Part model, mm, in its own coordinate system. A direction names the side the tool comes from. Coordinates: 2 decimals unless noted, no trailing zeros. Write each loop counter-clockwise with the first axis right and the second up, starting at its lowest first coordinate (ties: lowest second). Pieces come first, ordered by that corner, then holes. Notation, with made-up numbers: (1, -37) - (21, -37) arc R17 ccw to (21, -14) - close; hole circle Ø4 at (19.25, 14). An arc over 180 degrees is marked (long way). Use a Markdown table: item, result.
```python
from build123d import *

# Parameters (mm, degrees)
SKETCH1_W           = 900
SKETCH1_H           = 50
BOSS_EXTRUDE1_DEPTH = 200
BOSS_EXTRUDE2_START = -82
SKETCH4_R           = 20
SKETCH4_R_2         = 15.875
BOSS_EXTRUDE2_DEPTH = 36
SKETCH8_W           = 25
SKETCH8_H           = 252.75
BOSS_EXTRUDE3_DEPTH = 25
FILLET1_R           = 50
SKETCH9_R           = 15.875
BOSS_EXTRUDE4_DEPTH = 18


with BuildPart() as part:
    # Sketch1 → Boss-Extrude1 (new body)
    with BuildSketch(Plane.XY):
        with Locations((370.54501266, -26.765800796)):
            Rectangle(SKETCH1_W, SKETCH1_H)
    extrude(amount=BOSS_EXTRUDE1_DEPTH)

    # Sketch4 → Boss-Extrude2 (add)
    # profile 1 of 2: a face of its own
    with BuildSketch(Plane(origin=(0, 0, 0), x_dir=(-1, 0, 0), z_dir=(0, 0, -1)).offset(BOSS_EXTRUDE2_START)):
        with BuildLine():
            Line((79.45498734, -16.105071334), (79.45498734, -26.765800796))
            Line((79.45498734, -26.765800796), (79.45498734, -39.539290307))
            Line((79.45498734, -39.539290307), (107.065446551, -39.539290307))
            ThreePointArc((107.065446551, -39.539290307), (102.497605949, -28.070763635), (105.53314207, -16.105071334))
            Line((105.53314207, -16.105071334), (79.45498734, -16.105071334))
        make_face()
    # profile 2 of 2: a face of its own
    with BuildSketch(Plane(origin=(0, 0, 0), x_dir=(-1, 0, 0), z_dir=(0, 0, -1)).offset(BOSS_EXTRUDE2_START)):
        with Locations((122.45498734, -26.765800796)):
            Circle(SKETCH4_R)
        with Locations((122.45498734, -26.765800796)):
            Circle(SKETCH4_R_2, mode=Mode.SUBTRACT)
    extrude(amount=-BOSS_EXTRUDE2_DEPTH)

    # Sketch8 → Boss-Extrude3 (add, symmetric)
    with BuildSketch(Plane.XY.offset(100)):
        with Locations((349.31501266, 124.609199204)):
            Rectangle(SKETCH8_W, SKETCH8_H)
    extrude(amount=BOSS_EXTRUDE3_DEPTH, both=True)

    # Fillet1
    fillet1_edges = [part.edges().sort_by_distance(p)[0] for p in [
        (349.31501266, -1.765800796, 75),
        (336.81501266, -1.765800796, 100),
        (361.81501266, -1.765800796, 100),
        (349.31501266, -1.765800796, 125),
    ]]
    fillet(fillet1_edges, radius=FILLET1_R)

    # Sketch9 → Boss-Extrude4 (add, symmetric)
    with BuildSketch(Plane.XY.offset(100)):
        with BuildLine():
            Line((343.39732273, 250.984199204), (355.564186934, 250.984199204))
            Line((355.564186934, 250.984199204), (355.564186934, 261.985572388))
            ThreePointArc((355.564186934, 261.985572388), (349.141025878, 300.983442405), (343.39732273, 261.879724705))
            Line((343.39732273, 261.879724705), (343.39732273, 250.984199204))
        make_face()
        with Locations((349.31501266, 280.984199204)):
            Circle(SKETCH9_R, mode=Mode.SUBTRACT)
    extrude(amount=BOSS_EXTRUDE4_DEPTH, both=True)


solid = part.part
```
Item 1: Two-plate mould, pull along Y, no slides. Class faces 4 (the face through (364, -51.766, 99)), 5 (the face through (315.042, 6.964, 101.05)), 6 (the face through (351, 265, 82)), 7 (the face through (361.815, 148, 100)): pulls with the +Y half, pulls with the -Y half, needs draft (parallel to the pull), parting line crosses it, or undercut.
From the geometry:
| item | result |
|---|---|
| face 4 | pulls with the -Y half |
| face 5 | undercut |
| face 6 | needs draft |
| face 7 | undercut |
Item 2: Drill centre lines: probe 1 along Y at (x, z) = (232, 110); probe 2 along X at (y, z) = (223.5, 77.5); probe 3 along Y at (x, z) = (388.5, 77). Where is each one in solid material? Low to high.
From the geometry:
| item | result |
|---|---|
| probe 1 | -51.77 to -1.77 |
| probe 2 | 336.82 to 361.82 |
| probe 3 | -51.77 to 4 |
Item 3: Band-saw the part on B-B, the plane y = 242.5. Give the cut face in (x, z).
From the geometry:
| item | result |
|---|---|
| outline | (336.82, 75) - (361.82, 75) - (361.82, 125) - (336.82, 125) - close |
Item 4: Band-saw the part on D-D, the plane z = 141.5. Give the cut face in (x, y), then the cut area to 3 significant figures.
From the geometry:
| item | result |
|---|---|
| outline | (-79.45, -51.77) - (820.55, -51.77) - (820.55, -1.77) - (411.82, -1.77) arc R50 cw to (378.32, 11.12) - (320.32, 11.12) arc R50 cw to (286.82, -1.77) - (-79.45, -1.77) - close |
| area | 46,000 mm^2 |
Item 5: Drop flat-ended pins along their axis: P1, Ø12.5, axis at x = 350.5, y = 140.5, coming from the +Z side; P2, Ø19, axis at x = 349.32, y = 280.98, coming from the +Z side; P3, Ø8, axis at x = -92.5, z = 103.5, coming from the +Y side; P4, Ø5.5, axis at y = 255, z = 95.5, coming from the -X side. Give the stop position or say it passes through.
From the geometry:
| item | result |
|---|---|
| P1 | z = 125 |
| P2 | through |
| P3 | y = -16.11 |
| P4 | x = 343.4 |
Item 6: Which spindle directions (+Z, -Z, +X, -X, +Y, -Y) get a long thin tool onto all of the face, cutting with end or side? Do faces 1 (the face through (383.588, 6.964, 101.05)), 2 (the face through (-104, -26, 82)), 3 (the face through (-104, -26, 118)). Say none if no direction does.
From the geometry:
| item | result |
|---|---|
| face 1 | +Z, -Z, +X |
| face 2 | -Z, -X, +Y, -Y |
| face 3 | +Z, -X, +Y, -Y |
Item 7: Band-saw the part on A-A, the plane z = 50. Give the cut face in (x, y), then the cut area to 3 significant figures.
From the geometry:
| item | result |
|---|---|
| outline | (-79.45, -51.77) - (820.55, -51.77) - (820.55, -1.77) - (411.82, -1.77) arc R50 cw to (386.82, 4.93) - (311.82, 4.93) arc R50 cw to (286.82, -1.77) - (-79.45, -1.77) - close |
| area | 45,600 mm^2 |
Item 8: Band-saw the part on C-C, the plane x = 0. Give the cut face in (y, z).
From the geometry:
| item | result |
|---|---|
| outline | (-51.77, 0) - (-1.77, 0) - (-1.77, 200) - (-51.77, 200) - close |
